Geometry check sheet. Reference: the model listing, model coordinates, mm. Face numbers are marked on the shaded views. A direction names the side the tool comes from. Round coordinates to 2 decimals unless told otherwise and drop trailing zeros. Order: outer loops, then holes, each group sorted by start corner. A loop starts at its lowest first (then second) coordinate and runs counter-clockwise, first axis right, second up. Notation, with made-up numbers: (0, 59.5) - (42, 59.5) arc R29 ccw to (42, 88.5) - close; hole circle Ø3 at (73.25, 25.25). An arc over 180 degrees is marked (long way). Return JSON: item names as keys, results as strings. Group by question number.
Q1. Sectioned sample at A-A, the plane z = -45. Record the cut outline in (x, y), then the cut area to 3 significant figures.
Q2. Material ranges on line 1 along Y through (x, z) = (-17.5, -45); line 2 along Y through (x, z) = (-5.25, -45); line 3 along Z through (x, y) = (-12.5, 6.5), recorded low to high.
Q3. Draft check along Z on the marked faces 1, 2 and 3. Enter one of: pulls with the +Z half, pulls with the -Z half, needs draft (parallel to the pull), parting line crosses it, or undercut.
Q4. Gauge pin test, flat ends, axial feed: pin 1 Ø3 at (x, y) = (-17, 19) entering from -Z; pin 2 Ø8 at (x, z) = (-12.5, -9.41) entering from +Y; pin 3 Ø6 at (x, z) = (-12.5, -80.59) entering from +Y. Record the tip position at first contact, or that the pin passes through.
Q5. Sectioned sample at D-D, the plane x = -16.25. Give the number of separate pieces and of enclosed holes in the cut face, then the cut area to 3 significant figures.
Q6. Tool access check on the marked faces 4 and 5. Record the directions out of +Z, -Z, +X, -X, +Y, -Y that give a thin tool (end or side, any length) a straight path to the whole face; none if there is none.
Q7. Sectioned sample at C-C, the plane x = -12.75. Record the cut outline in (y, z), then the cut area to 3 significant figures.
Q8. Sectioned sample at B-B, the plane y = 7.5. Record the cut outline in (x, z).
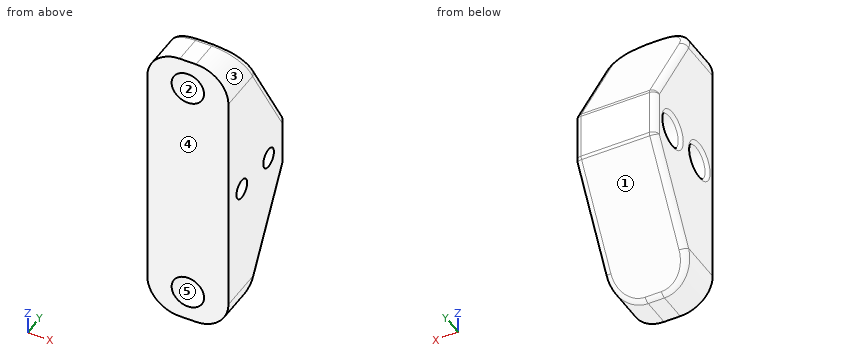
Autodesk Inventor part; units mm, degrees
ref_plane "YZ Plane" through (0, 0, 0) normal (1, 0, 0) x (0, 1, 0)
ref_plane "XZ Plane" through (0, 0, 0) normal (0, 1, 0) x (-1, 0, 0)
ref_plane "XY Plane" through (0, 0, 0) normal (0, 0, 1) x (1, 0, 0)
sketch "Sketch1" plane through (0, 0, 0) normal (0, 1, 0) x (-1, 0, 0)
  line L0 (0, 0) -> (25, 0)
  line L1 (25, 0) -> (25, -90)
  line L2 (25, -90) -> (0, -90)
  line L3 (0, -90) -> (0, 0)
  dimension "d0" = 25
  dimension "d1" = 90
extrude "Extrusion1" add sketch "Sketch1" along normal blind 10
sketch "Sketch2" plane through (0, 10, 0) normal (0, 1, 0) x (1, 0, 0)
  line L0 (-25, 90) -> (-25, 0)
  line L1 (0, 0) -> (0, 90)
  line L2 (-25, 37.5) -> (0, 37.5)
  line L3 (0, 37.5) -> (0, 52.5)
  line L4 (0, 52.5) -> (-25, 52.5)
  line L5 (-25, 52.5) -> (-25, 37.5)
  line L6 (-25, 0) -> (0, 0)
  point P0 (-25, 80)
  point P1 (-25, 10)
  point P2 (0, 10)
  point P3 (0, 80)
  point P4 (-15, 0)
  point P5 (-10, 0)
  point P6 (0, 37.5)
  dimension "d5" = 15
  dimension "d6" = 37.5
extrude "Extrusion2" add sketch "Sketch2" along normal blind 22 contours L4 L1 L2 L0
sketch "Sketch3" plane through (-25, 10, -37.5) normal (0, 0, 1) x (1, 0, 0)
  point P0 (25, -10)
sketch "Sketch5" plane through (0, 0, 0) normal (1, 0, 0) x (0, 0, -1)
  line L0 (37.5, 10) -> (37.5, 32)
  line L1 (0, 10) -> (37.5, 10)
  line L2 (37.5, 32) -> (0, 10)
  line L3 (37.5, 32) -> (52.5, 32)
  line L4 (52.5, 32) -> (90, 10)
  line L5 (90, 10) -> (52.5, 10)
  line L6 (52.5, 10) -> (90, 10)
  line L7 (52.5, 10) -> (52.5, 32)
  line L8 (52.5, 32) -> (52.5, 10)
  point P0 (0, 0)
extrude "Extrusion3" add sketch "Sketch5" against normal blind 25
fillet "Fillet2" radius 10 4 edges at (-25, 5, 0) (0, 5, 0) (-25, 5, -90) (0, 5, -90)
fillet "Fillet3" radius 2 14 edges at (-12.5, 32, -52.5) (-12.5, 32, -37.5) (0, 32, -45) (-2.9289, 11.7183, -87.0711) (-12.5, 10, -90) (-22.0711, 11.7183, -87.0711) (-25, 23.9333, -66.25) (0, 23.9333, -66.25) (-2.9289, 11.7183, -2.9289) (-12.5, 10, 0) (-22.0711, 11.7183, -2.9289) (-25, 23.9333, -23.75) (0, 23.9333, -23.75) (-25, 32, -45)
sketch "Sketch6" plane through (-25, 0, -80) normal (-1, 0, 0) x (0, 0, 1)
  line L0 (28.0434, 30) -> (41.9566, 30)
  line L1 (35, 30) -> (35, 15)
  line L2 (70, 0) -> (0, 0)
  line L3 (35, 30) -> (35, 0)
  line L4 (35, 15) -> (35, 0)
  circle A0 centre (35, 7.5) radius 3
  circle A1 centre (35, 22.5581) radius 3
  point P0 (80, 0)
  point P1 (35, 22.5)
  dimension "d13" = 6
  dimension "d14" = 7.5
  dimension "d15" = 6
extrude "Extrusion4" cut sketch "Sketch6" against normal blind 25
sketch "Sketch7" plane through (-25, 0, -80) normal (-1, 0, 0) x (0, 0, 1)
  circle A0 centre (35, 22.5581) radius 3
  line L0 (35, 25.5581) -> (35, 19.5581)
  circle A1 centre (35, 22.5581) radius 5
  circle A2 centre (35, 7.5) radius 3
  line L1 (35, 10.5) -> (35, 4.5)
  circle A3 centre (35, 7.5) radius 5
  point P0 (80, 0)
  dimension "d18" = 10
  dimension "d19" = 10
extrude "Extrusion5" cut sketch "Sketch7" against normal blind 10
fillet "Fillet4" radius 1 2 edges at (-25, 22.5581, -50) (-25, 7.5, -50)
sketch "Sketch8" plane through (0, 0, 0) normal (0, -1, 0) x (1, 0, 0)
  line L0 (-10, -90) -> (-15, -90)
  line L1 (-12.5, -90) -> (-12.5, 0)
  line L2 (-15, 0) -> (-10, 0)
  circle A0 centre (-12.5, -80.5935) radius 5
  circle A1 centre (-12.5, -9.4065) radius 5
  point P0 (0, 0)
  point P1 (-12.5, -45)
  point P2 (-12.5, -4.4065)
  point P3 (-12.5, -14.4065)
  point P4 (-12.5, -75.5935)
  point P5 (-12.5, -85.5935)
  dimension "d23" = 71.187
  dimension "d24" = 10
  dimension "d25" = 10
  dimension "d26" = 35.5935
extrude "Extrusion6" cut sketch "Sketch8" against normal blind 10
properties part number "Triangle_Bracket"
Reply:
{
 "1": {"outline": "(-25, 0) - (0, 0) - (0, 4.5) - (-15, 4.5) - (-15, 2.5) - (-24, 2.5) arc R1 ccw to (-25, 1.5) - close; (-25, 13.5) arc R1 ccw to (-24, 12.5) - (-15, 12.5) - (-15, 10.5) - (0, 10.5) - (0, 19.56) - (-15, 19.56) - (-15, 17.56) - (-24, 17.56) arc R1 ccw to (-25, 16.56) - close; (-25, 28.56) arc R1 ccw to (-24, 27.56) - (-15, 27.56) - (-15, 25.56) - (0, 25.56) - (0, 30) arc R2 ccw to (-2, 32) - (-23, 32) arc R2 ccw to (-25, 30) - close", "area": "417 mm^2"},
 "2": {"line 1": "0 to 2.5, 12.5 to 17.56, 27.56 to 32", "line 2": "0 to 4.5, 10.5 to 19.56, 25.56 to 32", "line 3": "-90 to -85.59, -75.59 to -47.83, -42.17 to -14.41, -4.41 to 0"},
 "3": {"face 1": "pulls with the -Z half", "face 2": "undercut", "face 3": "pulls with the +Z half"},
 "4": {"pin 1": "z = -77.22", "pin 2": "y = 17.87", "pin 3": "y = 17.28"},
 "5": {"separate pieces": "1", "enclosed holes": "2", "area": "1,760 mm^2"},
 "6": {"face 4": "+Z, -Z, +X, -X, -Y", "face 5": "-Y"},
 "7": {"outline": "(0, -90) - (8.85, -90) arc R2 ccw to (10.58, -89.01) - (31.73, -52.97) arc R2 ccw to (32, -51.96) - (32, -38.04) arc R2 ccw to (31.73, -37.03) - (10.58, -0.99) arc R2 ccw to (8.85, 0) - (0, 0) - (0, -4.41) - (10, -4.41) - (10, -14.4) - (0, -14.4) - (0, -75.6) - (10, -75.6) - (10, -85.59) - (0, -85.59) - close; hole circle Ø6 at (7.5, -45); hole circle Ø6 at (22.56, -45)", "area": "1,800 mm^2"},
 "8": {"outline": "(-25, -80) arc R10 ccw to (-15, -90) - (-10, -90) arc R10 ccw to (0, -80) - (0, -48) - (-15, -48) - (-15, -50) - (-24, -50) arc R1 ccw to (-25, -51) - close; (-25, -39) arc R1 ccw to (-24, -40) - (-15, -40) - (-15, -42) - (0, -42) - (0, -10) arc R10 ccw to (-10, 0) - (-15, 0) arc R10 ccw to (-25, -10) - close; hole circle Ø10 at (-12.5, -80.59); hole circle Ø10 at (-12.5, -9.41)"}
}
